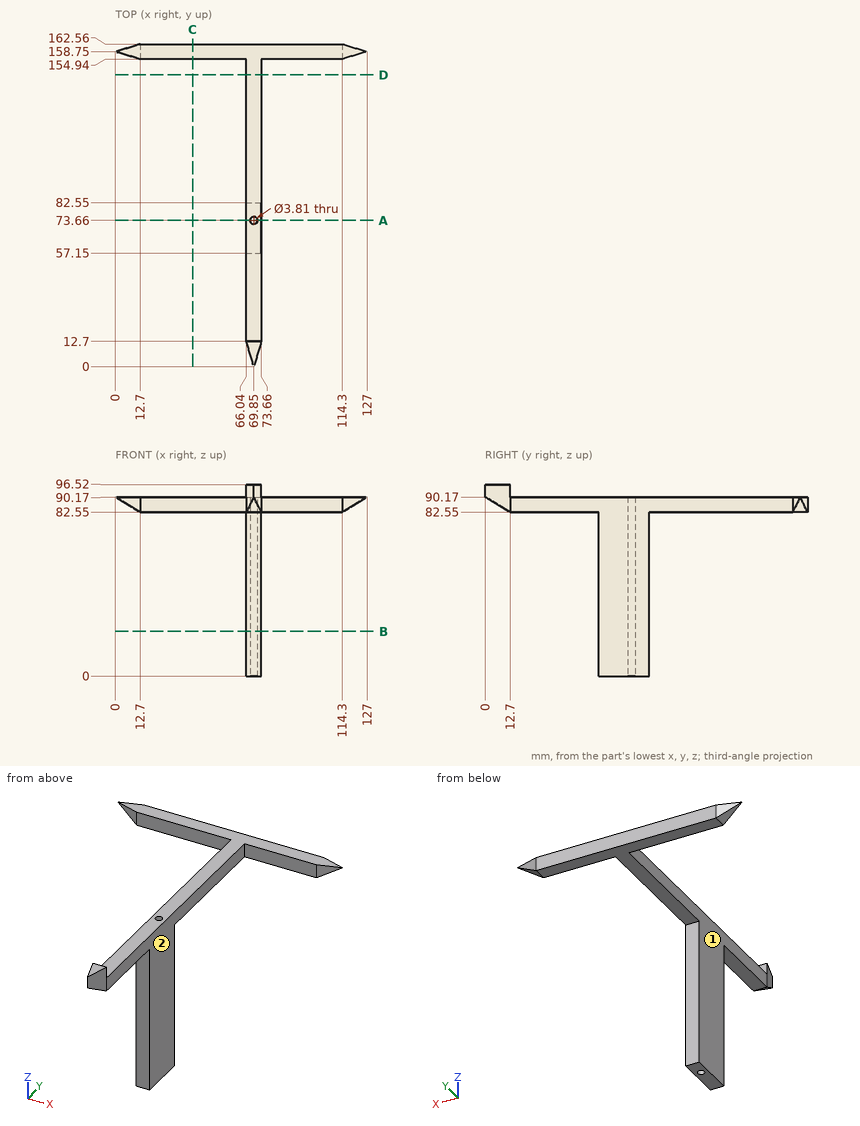
Can you work these out from the drawing? Everything is in mm from the part's minimum corner. A direction names the side the tool comes from. Round coordinates to 2 decimals unless told otherwise and drop trailing zeros. Order: outer loops, then holes, each group sorted by start corner. A loop starts at its lowest first (then second) coordinate and runs counter-clockwise, first axis right, second up. Notation, with made-up numbers: (70, 70) - (90, 70) arc R29 cw to (90, 101) - close; hole circle Ø4 at (-17, 30). An arc over 180 degrees is marked (long way). Answer in a Markdown table with one row per item.
(1) Which directions (+Z, -Z, +X, -X, +Y, -Y) give clear straight access to the entire face, cutting with the end or side of a thin tool? Please do the marked faces 1 and 2.
From the geometry:
| item | result |
|---|---|
| face 1 | +Z, -Z, -X, -Y |
| face 2 | +Z, -Z, +X, -Y |
(2) Suppose I cut it at D-D, the plane y = 147. Please give me the cut outline in (x, z), plus the area to 3 significant figures.
From the geometry:
| item | result |
|---|---|
| outline | (66.04, 82.55) - (73.66, 82.55) - (73.66, 90.17) - (66.04, 90.17) - close |
| area | 58.1 mm2 |
(3) Suppose I cut it at C-C, the plane x = 39. Please give me the cut outline in (y, z), plus the area to 3 significant figures.
From the geometry:
| item | result |
|---|---|
| outline | (154.94, 82.55) - (162.56, 82.55) - (162.56, 90.17) - (154.94, 90.17) - close |
| area | 58.1 mm2 |
(4) Suppose I cut it at B-B, the plane z = 22.5. Please give me the cut outline in (x, y) (3 decimals), plus the area to 3 significant figures.
From the geometry:
| item | result |
|---|---|
| outline | (66.04, 57.15) - (73.66, 57.15) - (73.66, 82.55) - (66.04, 82.55) - close; hole circle Ø3.81 at (69.85, 73.66) |
| area | 182 mm2 |
(5) Suppose I cut it at A-A, the plane y = 73.66. Please give me the cut outline in (x, z) (3 decimals).
From the geometry:
| item | result |
|---|---|
| outline | (66.04, 0) - (67.945, 0) - (67.945, 90.17) - (66.04, 90.17) - close; (71.755, 0) - (73.66, 0) - (73.66, 90.17) - (71.755, 90.17) - close |
(6) Please list where these lines run through material, in increasing order: L1, parallel to Y at x = 69.85, z = 24.5 (3 decimals); L2, parallel to X at y = 73.66, z = 51.5 (3 decimals); L3, parallel to X at y = 71, z = 67. Write a range as from..to.
From the geometry:
| item | result |
|---|---|
| L1 | y = 57.15..71.755, 75.565..82.55 |
| L2 | x = 66.04..67.945, 71.755..73.66 |
| L3 | x = 66.04..73.66 |
(7) For P1, Ø4, axis at x = 101, z = 86.5, coming from the -Y side; P2, Ø6, axis at x = 69.85, y = 73.66, coming from the +Z side; P3, Ø12, axis at y = 140, z = 83.5, coming from the -X side; P4, Ø4, axis at y = 36.5, z = 80, coming from the -X side, each with a flat end and sliding along its axis, tell me the tip position at first contact or that it passes through.
From the geometry:
| item | result |
|---|---|
| P1 | stops at y = 154.94 |
| P2 | stops at z = 90.17 |
| P3 | stops at x = 66.04 |
| P4 | passes through |
